Verification items for this drawing (mm, ordinates from the low corner). A direction names the side the tool comes from. Round coordinates to 2 decimals unless told otherwise and drop trailing zeros. Loops run counter-clockwise (first coordinate to the right, second up) from the corner with the lowest first, then second, coordinate; pieces in that order, holes last. Notation, with made-up numbers: (37.25, 87) - (64.25, 87) arc R13 ccw to (64.25, 108) - close; hole circle Ø9 at (36, -3). An arc over 180 degrees is marked (long way). Answer in a Markdown table with one row per item. Add a question column.
(1) Cross-section at B-B on z = 98. Enter the section's corners in (x, y) (1 decimal), then the cut area to 3 significant figures.
(2) Cross-section at C-C on x = 81. Enter the section's corners in (y, z) (1 decimal), then the cut area to 3 significant figures.
(3) Cross-section at A-A on y = 15. Enter the section's corners in (x, z) (1 decimal).
(4) Access from +Z, -Z, +X, -X, +Y, -Y to the whole of each face (thin tool, end or side, straight path). Record for the marked faces 1, 2, 3, 4 and 5.
(5) Gauge pin test, flat ends, axial feed: pin 1 (4 mm diameter, centred on x = 7, y = 48, fed in from -Z); pin 2 (1 mm diameter, centred on y = 35, z = 89, fed in from +X); pin 3 (1.5 mm diameter, centred on x = 82, z = 88, fed in from -Y). Record the tip position at first contact, or that the pin passes through.
(6) Cross-section at D-D on z = 65.5. Enter the section's corners in (x, y) (1 decimal), then the cut area to 3 significant figures.
(7) Mould release check, pull along Z, two halves, no side actions. Record for the marked faces 6, 7 and 8: +Z half, -Z half, draft (parallel to the pull), parting line (faces both ways), or undercut.
(8) Thickness scan on line 1 along X through (y, z) = (46, 33); line 2 along Z through (x, y) = (69, 25) (1 decimal); line 3 along Z through (x, y) = (38, 51) (1 decimal). Record the ranges inside material, lowest first.
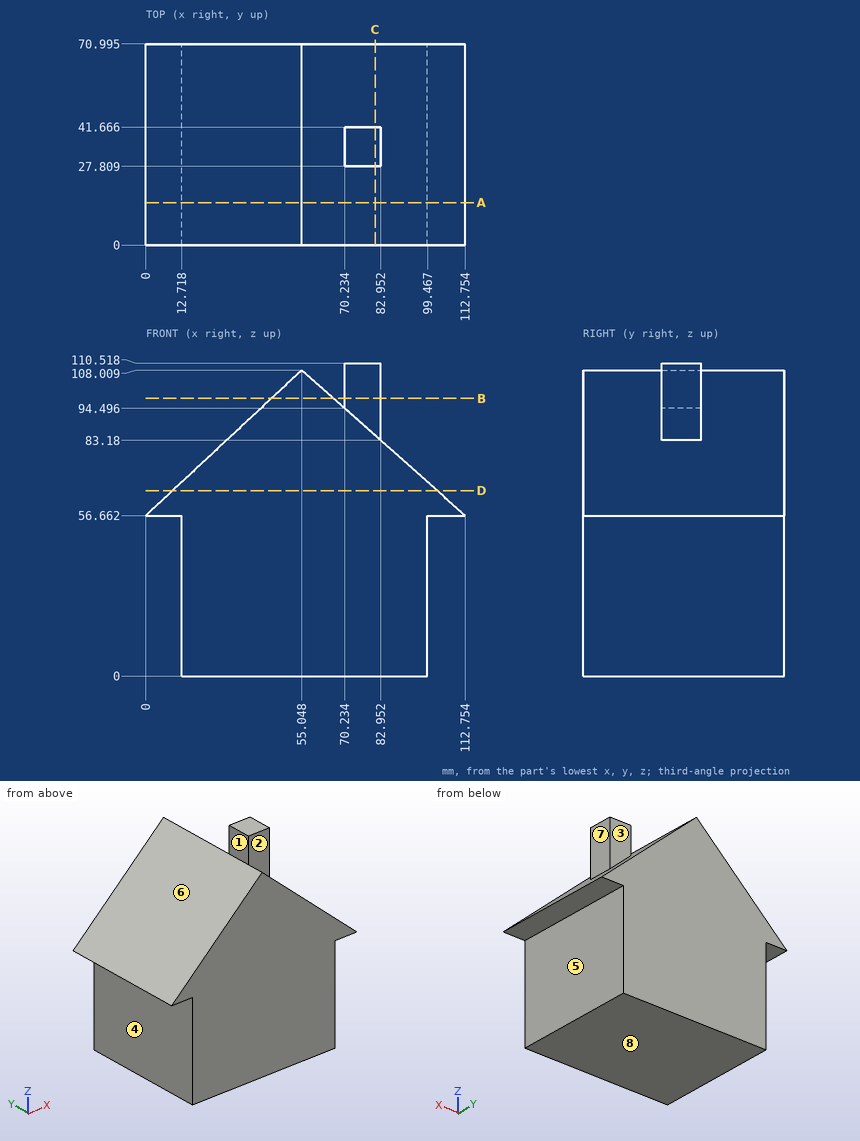
Answers:
| question | item | result |
|---|---|---|
| 1 | outline | (44.3, 0) - (66.3, 0) - (66.3, 71) - (44.3, 71) - close; (70.2, 27.8) - (83, 27.8) - (83, 41.7) - (70.2, 41.7) - close |
| 1 | area | 1,740 mm^2 |
| 2 | outline | (0, 0) - (71, 0) - (71, 84.9) - (41.7, 84.9) - (41.7, 110.5) - (27.8, 110.5) - (27.8, 84.9) - (0, 84.9) - close |
| 2 | area | 6,380 mm^2 |
| 3 | outline | (0, 56.7) - (12.7, 56.7) - (12.7, 0) - (99.5, 0) - (99.5, 56.7) - (112.8, 56.7) - (55, 108) - close |
| 4 | face 1 | +Z, +Y, -Y |
| 4 | face 2 | +Z, +X, -Y |
| 4 | face 3 | +Z, +X, +Y |
| 4 | face 4 | -Z, -X, +Y, -Y |
| 4 | face 5 | -Z, +X, +Y, -Y |
| 5 | pin 1 | stops at z = 56.66 |
| 5 | pin 2 | stops at x = 82.95 |
| 5 | pin 3 | stops at y = 27.81 |
| 6 | outline | (9.5, 0) - (102.8, 0) - (102.8, 71) - (9.5, 71) - close |
| 6 | area | 6,630 mm^2 |
| 7 | face 6 | +Z half |
| 7 | face 7 | draft |
| 7 | face 8 | -Z half |
| 8 | line 1 | x = 12.72 to 99.47 |
| 8 | line 2 | z = 0 to 95.6 |
| 8 | line 3 | z = 0 to 92.1 |
